Source: CAD feature listing. Evaluate the final solid. Frame: model axes, mm. A direction names the side the tool comes from. Give positions to 0.01 mm unless a question says otherwise; leave off trailing zeros. Write each loop counter-clockwise with the first axis right and the second up, starting at its lowest first coordinate (ties: lowest second). Pieces come first, ordered by that corner, then holes. Notation, with made-up numbers: M 41.25,11 L 76.25,11 A8 ccw 76.25,21 Z; hole C -22,7.25 d10. An arc over 180 degrees is marked long. Return JSON: item names as keys, results as strings.
```python
from build123d import *

# Parameters (mm, degrees)
SM_BASE_FLANGE_1_DEPTH = 160
OTHER_START            = -160
OTHER_1_DEPTH          = 320
OTHER_1_2_DEPTH        = 320
SKETCH_4_R             = 1.6
CUT_EXTRUDE_1_DEPTH    = 2


# Read off the part's stored shape, not the designer's step: 绘制的折弯1
# Sheet-metal steps are written as plain solids
with BuildPart() as part:
    # Sketch 1 → 基体-法兰1 (new, symmetric)
    with BuildSketch(Plane(origin=(0, 0, 0), x_dir=(0, 0, -1), z_dir=(1, 0, 0))):
        with BuildLine():
            Line((-32, 23), (0, 23))
            ThreePointArc((0, 23), (23, 0), (0, -23))
            Line((0, -23), (-19, -23))
            Line((-19, -23), (-19, -22))
            Line((-19, -22), (0, -22))
            ThreePointArc((0, -22), (22, 0), (0, 22))
            Line((0, 22), (-32, 22))
            Line((-32, 22), (-32, 23))
        make_face()
    extrude(amount=SM_BASE_FLANGE_1_DEPTH, both=True)

    # Other 1 outline → Other 1 (cut)
    with BuildSketch(Plane.YZ.offset(OTHER_START)):
        with BuildLine():
            ThreePointArc((22, 15.2634), (22.271171885, 16.195226164), (23, 16.83604109))
            Line((23, 16.83604109), (23, 32))
            Line((23, 32), (22, 32))
            Line((22, 32), (22, 15.2634))
        make_face()
    extrude(amount=OTHER_1_DEPTH, mode=Mode.SUBTRACT)

    # Other 1 2 outline → Other 1 2 (add)
    with BuildSketch(Plane.YZ.offset(OTHER_START)):
        with BuildLine():
            ThreePointArc((23, 15.2634), (23.215745145, 15.784254855), (23.7366, 16))
            Line((23.7366, 16), (38.530753262, 16))
            Line((38.530753262, 16), (38.530753262, 17))
            Line((38.530753262, 17), (23.7366, 17))
            ThreePointArc((23.7366, 17), (23.359286442, 16.958514757), (23, 16.83604109))
            Line((23, 16.83604109), (23, 15.2634))
        make_face()
    extrude(amount=OTHER_1_2_DEPTH)

    # 草图4 → 切除-拉伸1 (cut)
    with BuildSketch(Plane(origin=(0, 0, 16), x_dir=(-1, 0, 0), z_dir=(0, 0, -1))):
        with Locations(Location((0, 31.530753262, 0), (0, 0, 90))):
            Circle(SKETCH_4_R)
        with Locations(Location((145, 31.530753262, 0), (0, 0, 90))):
            Circle(SKETCH_4_R)
        with Locations(Location((65, 31.530753262, 0), (0, 0, 90))):
            Circle(SKETCH_4_R)
        with Locations(Location((-145, 31.530753262, 0), (0, 0, 90))):
            Circle(SKETCH_4_R)
        with Locations(Location((-65, 31.530753262, 0), (0, 0, 90))):
            Circle(SKETCH_4_R)
    extrude(amount=-CUT_EXTRUDE_1_DEPTH, mode=Mode.SUBTRACT)


solid = part.part
```
1) Contact query for flat-ended pins moving along their axis: pin 1 Ø16.5 at (x, y) = (-68.5, 35) entering from +Z; pin 2 Ø3 at (x, z) = (42.5, 14) entering from +Y; pin 3 Ø3 at (x, y) = (145, 31.53) entering from +Z; pin 4 Ø4 at (x, z) = (90.5, -6) entering from +Y. Output: stop coordinate, or through.
Numbers:
{"pin 1": "stops at z = 17", "pin 2": "stops at y = 23.04", "pin 3": "passes through", "pin 4": "stops at y = 22.65"}
2) Line query: line 1 (Y direction, x = -59, z = 10); line 2 (Y direction, x = 145, z = 16.55); line 3 (Z direction, x = 101, y = -0.5). Output: solid intervals per line, ascending. Write a range as [from, to].
Numbers:
{"line 1": "y = [-23, -22], [22, 23]", "line 2": "y = [-23, -22], [22.57, 29.93], [33.13, 38.53]", "line 3": "z = [-22.99, -21.99]"}
3) Cut plane A-A, the plane z = 9.5. Return the cut outline in (x, y).
Numbers:
{"outline": "M -160,-23 L 160,-23 L 160,-22 L -160,-22 Z; M -160,22 L 160,22 L 160,23 L -160,23 Z"}
4) Cut plane C-C, the plane z = -15. Return the cut outline in (x, y).
Numbers:
{"outline": "M -160,-17.44 L 160,-17.44 L 160,-16.09 L -160,-16.09 Z; M -160,16.09 L 160,16.09 L 160,17.44 L -160,17.44 Z"}
5) Set-up query: faces 1 (the face through (2, 22, 8)), 2 (the face through (-2, 31, 17)), 3 (the face through (160, -8, -21)). Return all of +Z, -Z, +X, -X, +Y, -Y with unobstructed straight access to the full face (end or side cutting, diameter ignored); none if empty.
Numbers:
{"face 1": "+Z, +X, -X", "face 2": "+Z, +X, -X, +Y", "face 3": "+Z, -Z, +X, +Y, -Y"}
6) Cut plane D-D, the plane y = 0. Return the cut outline in (x, z).
Numbers:
{"outline": "M -160,-23 L 160,-23 L 160,-22 L -160,-22 Z"}
7) Cut plane B-B, the plane x = -71. Return the cut outline in (y, z).
Numbers:
{"outline": "M -23,0 A23 ccw 23,0 L 23,15.26 A0.74 cw 23.74,16 L 38.53,16 L 38.53,17 L 23.74,17 A1.74 ccw 22,15.26 L 22,0 A22 cw -22,0 L -22,19 L -23,19 Z"}
8) Draft query along Y for faces 4 (the face through (2.24, 0.506, -22.994)), 5 (the face through (2, 23, 8)), 6 (the face through (2, -22, 10)), 7 (the face through (-2, 31, 16)). Return one class per face: released by +Y, released by -Y, zero draft, split by the parting line, or undercut.
Numbers:
{"face 4": "split by the parting line", "face 5": "released by +Y", "face 6": "undercut", "face 7": "zero draft"}
